The figure shows three views and two pictorial views of one solid part (mm, origin at its lowest corner). Answer the questions. Give positions to 0.01 mm unless a question says otherwise; leave off trailing zeros. Write each loop counter-clockwise with the first axis right and the second up, starting at its lowest first coordinate (ties: lowest second). Pieces come first, ordered by that corner, then holes. Notation, with made-up numbers: (23.5, -30) -> (49.5, -30) arc R9 ccw to (49.5, -15) -> close; hole circle Ø6 at (-13, 79). An arc over 180 degrees is marked (long way). Write item = value, one per line. Start each with the question number.
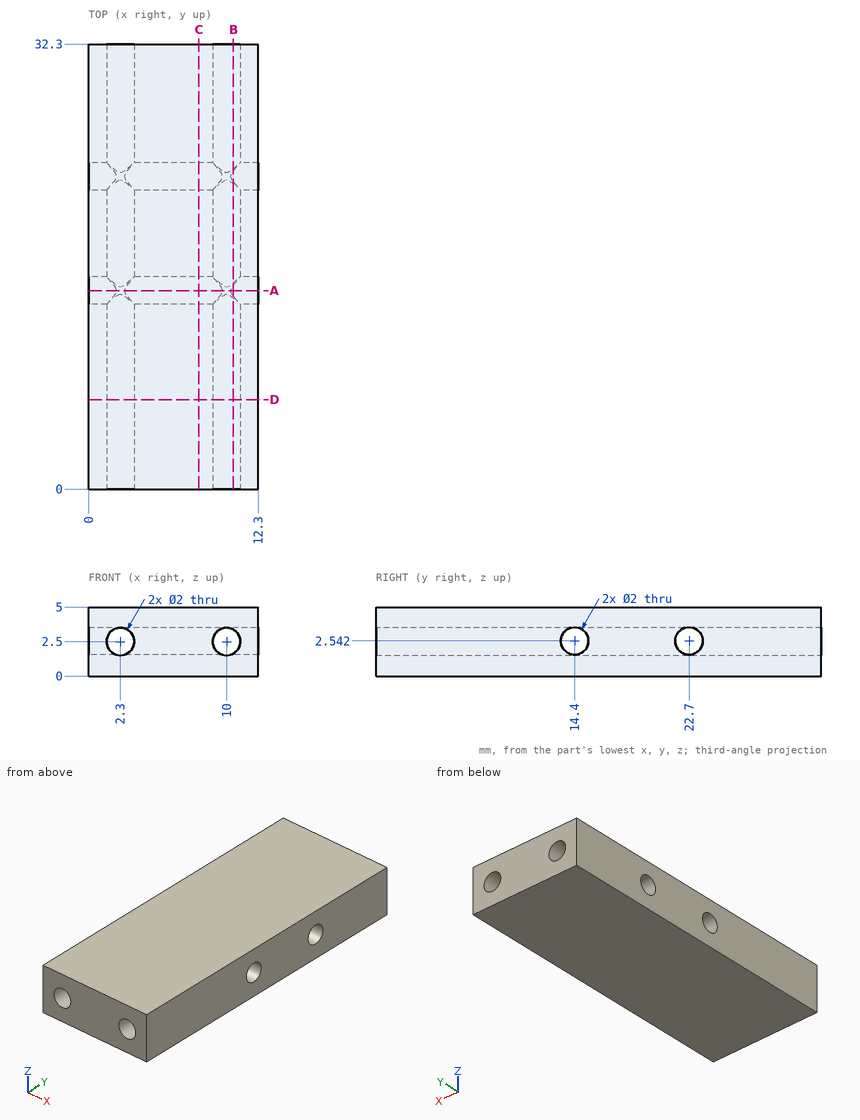
(1) A cutting plane is placed at A-A, the plane y = 14.4. Write down the section's boundary in (x, z).
(2) A cutting plane is placed at B-B, the plane x = 10.5. Write down the section's boundary in (y, z).
(3) Each of these flat-tipped pins is pushed along its axis until it touches: pin 1 (1.6 mm diameter, centred on y = 22.7, z = 2.54, fed in from -X); pin 2 (2.5 mm diameter, centred on y = 14.4, z = 2.54, fed in from +X). Where does it stop, or does it pass through?
(4) A cutting plane is placed at C-C, the plane x = 8. Write down the section's boundary in (y, z), then the cut area to 3 significant figures.
(5) A cutting plane is placed at D-D, the plane y = 6.5. Write down the section's boundary in (x, z).
(6) Find the intervals of material crossed by line 1 along X through (y, z) = (24, 2.5); line 2 along Y through (x, z) = (11.75, 2.45); line 3 along Y through (x, z) = (8, 3.1), in increasing order.
Results list:
q1.outline = (0, 0) -> (12.3, 0) -> (12.3, 1.54) -> (10.29, 1.54) arc R1 cw to (9.71, 1.54) -> (2.59, 1.54) arc R1 cw to (2.01, 1.54) -> (0, 1.54) -> close; (0, 3.54) -> (12.3, 3.54) -> (12.3, 5) -> (0, 5) -> close
q2.outline = (0, 0) -> (32.3, 0) -> (32.3, 1.63) -> (23.12, 1.63) arc R1 cw to (22.28, 1.63) -> (14.82, 1.63) arc R1 cw to (13.98, 1.63) -> (0, 1.63) -> close; (0, 3.37) -> (13.83, 3.37) arc R1 cw to (14.97, 3.37) -> (22.13, 3.37) arc R1 cw to (23.27, 3.37) -> (32.3, 3.37) -> (32.3, 5) -> (0, 5) -> close
q3.pin_1 = through
q3.pin_2 = 12.3
q4.outline = (0, 0) -> (32.3, 0) -> (32.3, 5) -> (0, 5) -> close; hole circle Ø2 at (14.4, 2.54); hole circle Ø2 at (22.7, 2.54)
q4.area = 155 mm²
q5.outline = (0, 0) -> (12.3, 0) -> (12.3, 5) -> (0, 5) -> close; hole circle Ø2 at (2.3, 2.5); hole circle Ø2 at (10, 2.5)
q6.line_1 = 0 to 1.3, 3.3 to 9, 11 to 12.3
q6.line_2 = 0 to 13.4, 15.4 to 21.7, 23.7 to 32.3
q6.line_3 = 0 to 13.57, 15.23 to 21.87, 23.53 to 32.3
